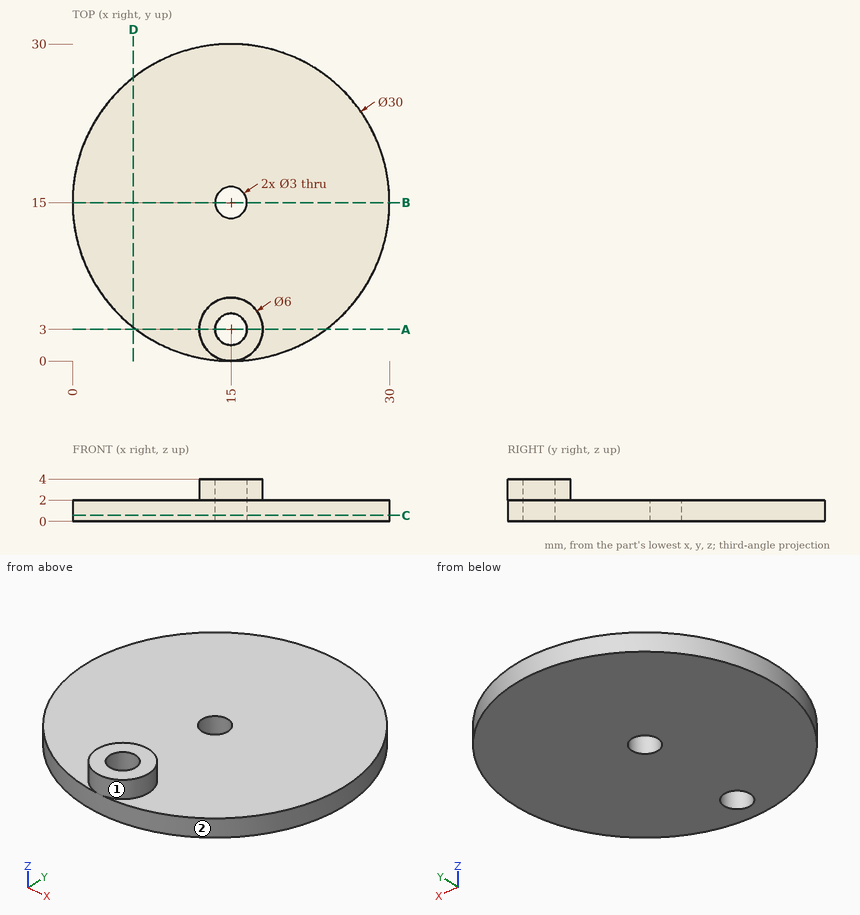
Could you check a few things on this drawing? It's one solid part, dimensions in mm from its lowest x, y, z. A direction names the side the tool comes from. Coordinates: 2 decimals unless noted, no trailing zeros. Order: outer loops, then holes, each group sorted by start corner. A loop starts at its lowest first (then second) coordinate and runs counter-clockwise, first axis right, second up. Notation, with made-up numbers: (-10, 55.5) -> (31, 55.5) arc R25 cw to (31, 91.5) -> close; hole circle Ø4 at (-29, 4.5). An arc over 180 degrees is marked (long way). One line per item, written item: value. Start each with the question number.
1) If I drill on L1, parallel to Y at x = 15, z = 1.2; L2, parallel to X at y = 3, z = 2.75; L3, parallel to Z at x = 13.25, y = 20.25, over which ranges is the centre line in solid material (lowest first)? Write a range as [from, to].
2) Imagine slicing it at B-B on y = 15. List the corners of the cut face in (x, z) for me.
3) Imagine slicing it at C-C on z = 0.55. List the corners of the cut face in (x, y) for me, plus the area to 3 significant figures.
4) Imagine slicing it at D-D on x = 5.75. List the corners of the cut face in (y, z) for me.
5) Which directions (+Z, -Z, +X, -X, +Y, -Y) give clear straight access to the entire face, cutting with the end or side of a thin tool? Please do the marked faces 1 and 2.
6) I'm going to push flat-ended pins straight in: pin 1 (1 mm diameter, centred on x = 19.5, z = 0.5, fed in from +Y); pin 2 (1.5 mm diameter, centred on y = 13.5, z = 1.5, fed in from +X); pin 3 (1 mm diameter, centred on x = 7.5, y = 18.5, fed in from +Z). Where does each tip first touch, or does it pass through?
7) Imagine slicing it at A-A on y = 3. List the corners of the cut face in (x, z) for me, plus the area to 3 significant figures.
Answer list:
1. L1: y = [0, 1.5], [4.5, 13.5], [16.5, 30]
1. L2: x = [12, 13.5], [16.5, 18]
1. L3: z = [0, 2]
2. outline: (0, 0) -> (13.5, 0) -> (13.5, 2) -> (0, 2) -> close; (16.5, 0) -> (30, 0) -> (30, 2) -> (16.5, 2) -> close
3. outline: circle Ø30 at (15, 15); hole circle Ø3 at (15, 3); hole circle Ø3 at (15, 15)
3. area: 693 mm2
4. outline: (3.19, 0) -> (26.81, 0) -> (26.81, 2) -> (3.19, 2) -> close
5. face 1: +Z
5. face 2: +Z, -Z
6. pin 1: stops at y = 29.46
6. pin 2: stops at x = 29.98
6. pin 3: stops at z = 2
7. outline: (6, 0) -> (13.5, 0) -> (13.5, 4) -> (12, 4) -> (12, 2) -> (6, 2) -> close; (16.5, 0) -> (24, 0) -> (24, 2) -> (18, 2) -> (18, 4) -> (16.5, 4) -> close
7. area: 36.0 mm2
